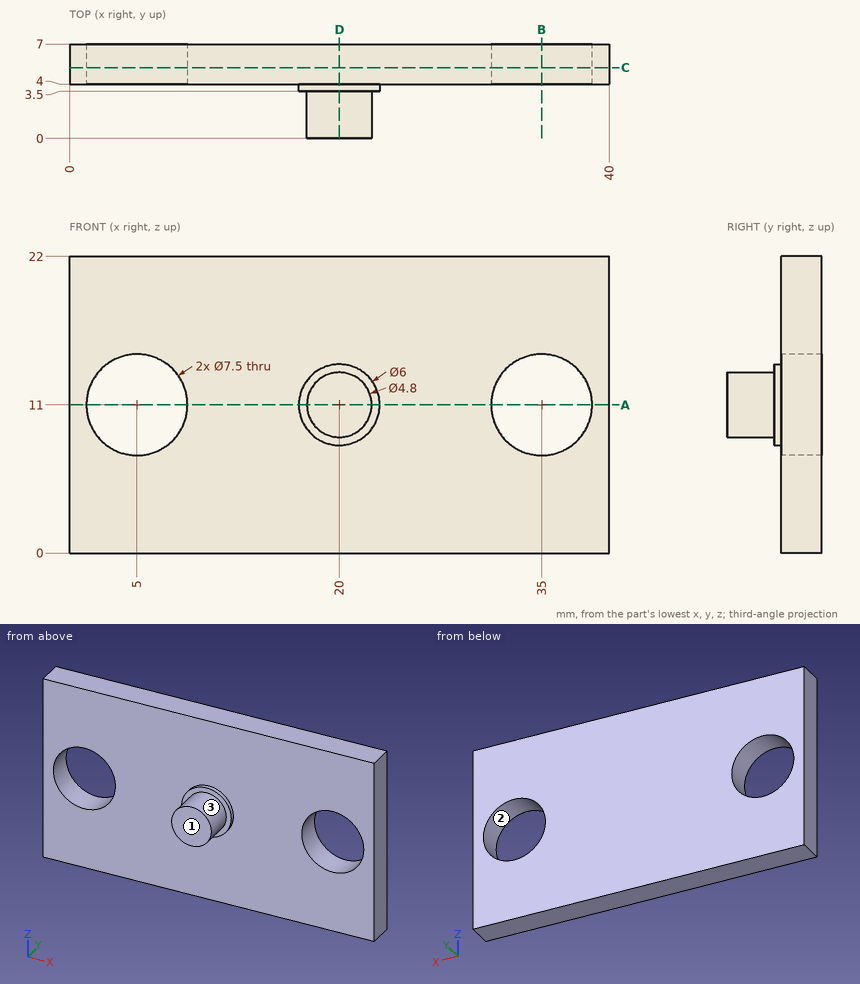
Part print with two shaded views. Sizes in mm from the minimum x, y, z corner. Coordinates: 2 decimals unless noted, no trailing zeros. Write each loop counter-clockwise with the first axis right and the second up, starting at its lowest first coordinate (ties: lowest second). Pieces come first, ordered by that corner, then holes.
1. Pull direction Z, two halves, no side cores. Call the marked faces 1, 2 and 3: released by +Z, released by -Z, zero draft, split by the parting line, or undercut.
Answer block:
face 1: zero draft
face 2: undercut
face 3: split by the parting line
2. Band-saw the part on B-B, the plane x = 35. Give the cut face in (y, z), and give its area (3 significant figures).
Answer block:
outline: (4, 0) - (7, 0) - (7, 7.25) - (4, 7.25) - close; (4, 14.75) - (7, 14.75) - (7, 22) - (4, 22) - close
area: 43.5 mm2
3. Band-saw the part on C-C, the plane y = 5.25. Give the cut face in (x, z), and give its area (3 significant figures).
Answer block:
outline: (0, 0) - (40, 0) - (40, 22) - (0, 22) - close; hole circle Ø7.5 at (5, 11); hole circle Ø7.5 at (35, 11)
area: 792 mm2
4. Drill centre lines: probe 1 along Z at (x, y) = (35, 5.05); probe 2 along Y at (x, z) = (7.5, 19); probe 3 along X at (y, z) = (4.5, 9.25). Where is each one in solid material? Low to high.
Answer block:
probe 1: z = 0 to 7.25, 14.75 to 22
probe 2: y = 4 to 7
probe 3: x = 0 to 1.68, 8.32 to 31.68, 38.32 to 40
5. Band-saw the part on A-A, the plane z = 11. Give the cut face in (x, y).
Answer block:
outline: (0, 4) - (1.25, 4) - (1.25, 7) - (0, 7) - close; (8.75, 4) - (17, 4) - (17, 3.5) - (17.6, 3.5) - (17.6, 0) - (22.4, 0) - (22.4, 3.5) - (23, 3.5) - (23, 4) - (31.25, 4) - (31.25, 7) - (8.75, 7) - close; (38.75, 4) - (40, 4) - (40, 7) - (38.75, 7) - close
6. Drop flat-ended pins along their axis: pin 1 (6 mm diameter, centred on x = 5, z = 11, fed in from -Y); pin 2 (6.5 mm diameter, centred on x = 26, z = 8.5, fed in from -Y). Give the stop position or say it passes through.
Answer block:
pin 1: passes through
pin 2: stops at y = 4
7. Band-saw the part on D-D, the plane x = 20. Give the cut face in (y, z).
Answer block:
outline: (0, 8.6) - (3.5, 8.6) - (3.5, 8) - (4, 8) - (4, 0) - (7, 0) - (7, 22) - (4, 22) - (4, 14) - (3.5, 14) - (3.5, 13.4) - (0, 13.4) - close
